Autodesk Inventor part; units mm, degrees
ref_plane "YZ Plane" through (0, 0, 0) normal (1, 0, 0) x (0, 1, 0)
ref_plane "XZ Plane" through (0, 0, 0) normal (0, 1, 0) x (-1, 0, 0)
ref_plane "XY Plane" through (0, 0, 0) normal (0, 0, 1) x (1, 0, 0)
sketch "Sketch1" plane through (0, 0, 0) normal (0, 1, 0) x (-1, 0, 0)
  line L0 (-0.0949, -0.0791) -> (-0.0949, -8.0791)
  circle A0 centre (-0.0949, -8.0791) radius 3
  line L1 (-0.0949, -0.0791) -> (-0.0949, 7.9209)
  circle A1 centre (-0.0949, 7.9209) radius 2.5
  circle A2 centre (-0.0949, 7.9209) radius 3.75
  circle A3 centre (-0.0949, -8.0791) radius 3.75
  line L2 (3.6551, 7.9209) -> (3.6551, -8.0791)
  line L3 (-3.8449, 7.9209) -> (-3.8449, -8.0791)
  line L4 (3.6551, 4.1709) -> (-3.8449, 4.1709)
  line L5 (3.6551, -4.3291) -> (-3.8449, -4.3291)
  point P0 (0, 0)
  dimension "d0" = 8
  dimension "d1" = 6
  dimension "d2" = 8
  dimension "d3" = 5
  dimension "d4" = 7.5
  dimension "d5" = 7.5
extrude "Extrusion1" add sketch "Sketch1" along normal blind 5 contours L1 L4 L2 L5 L0 | L0 L5 L3 L4 L1 | L5 L2 A3 | A3 | A3 L3 L5
sketch "Sketch2" plane through (-3.6551, 0, 4.1709) normal (0, 0, 1) x (1, 0, 0)
  line L0 (0, 5) -> (7.5, 5)
  line L1 (0, 0) -> (7.5, 0)
  line L2 (7.5, 0) -> (7.5, 5)
  line L3 (7.5, 5) -> (0, 5)
  line L4 (0, 5) -> (0, 0)
  line L5 (7.5, 5) -> (0, 5)
  line L6 (0, 5) -> (0, 0)
  line L7 (0, 0) -> (7.5, 0)
  line L8 (7.5, 0) -> (7.5, 5)
  line L9 (7.5, 5) -> (0, 0) construction
  line L10 (0, 5) -> (7.5, 0) construction
  circle A0 centre (3.75, 2.5) radius 1.5
  line L11 (6.25, 3.5) -> (1.25, 3.5)
  line L12 (1.25, 3.5) -> (1.25, 1.5)
  line L13 (1.25, 1.5) -> (6.25, 1.5)
  line L14 (6.25, 1.5) -> (6.25, 3.5)
  line L15 (6.25, 3.5) -> (1.25, 1.5) construction
  line L16 (1.25, 3.5) -> (6.25, 1.5) construction
  point P0 (3.6551, 0)
  point P1 (4.868, 1.5)
  point P2 (4.868, 3.5)
  point P3 (2.632, 3.5)
  point P4 (2.632, 1.5)
  dimension "d8" = 3
  dimension "d9" = 5
  dimension "d10" = 2
extrude "Extrusion2" cut sketch "Sketch2" against normal blind 8.5 contours A0 L13 L11 | A0 L11 L14 L13 | L11 A0 | A0 L13 | A0 L13 L12 L11
sketch "Sketch3" plane through (0, 5, 0) normal (0, 1, 0) x (1, 0, 0)
  line L0 (1.213, 4.3291) -> (2.5949, 4.3291)
  line L1 (-3.6551, -4.1709) -> (3.8449, -4.1709)
  point P0 (0, 0)
  dimension "d13" = 8.5
sketch "Sketch4" plane through (3.8449, 0, 4.1709) normal (1, 0, 0) x (0, 0, -1)
  line L0 (12.25, 0) -> (12.25, 5)
  circle A0 centre (12.25, 2.5) radius 1.5
  point P0 (4.1709, 0)
  dimension "d14" = 3
extrude "Extrusion3" add sketch "Sketch4" along normal mid plane 1.5
sketch "Sketch5" plane through (4.5949, 2.5, -8.0791) normal (1, 0, 0) x (0, 0, -1)
  line L0 (0, -2.5) -> (0, 2.5)
  circle A0 centre (0, 0) radius 1
  point P0 (-8.0791, -2.5)
  dimension "d17" = 2
extrude "Extrusion4" cut sketch "Sketch5" against normal blind 3.0875
properties part number "Link_OutsideV3"
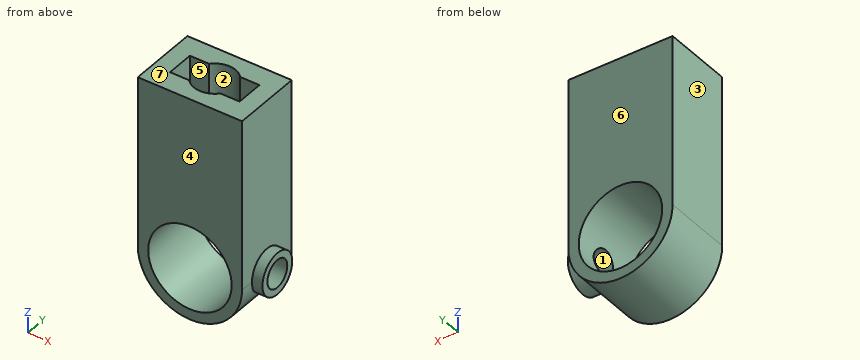
CAD build for the part. Positions are in the model's coordinates, mm. Face numbers are marked on the shaded views. A direction names the side the tool comes from. Coordinates: 2 decimals unless noted, no trailing zeros. Order: outer loops, then holes, each group sorted by start corner. A loop starts at its lowest first (then second) coordinate and runs counter-clockwise, first axis right, second up.
Item 1: Pin check, flat tips, straight feed: pin 1 Ø1.5 at (x, y) = (0.5, 2) entering from +Z; pin 2 Ø1.6 at (y, z) = (3, -1) entering from +X; pin 3 Ø1.5 at (x, z) = (-1.5, -8) entering from +Y. Stop position of each tip, or through.
Check sheet entries:
pin 1: stops at z = -4.33
pin 2: stops at x = 3.84
pin 3: passes through
Item 2: 3-axis set-ups, long thin cutter, end or side, ignore diameter. For the marked faces 1, 2 and 3: which of +Z, -Z, +X, -X, +Y, -Y reach the whole face in a straight line?
Check sheet entries:
face 1: +X
face 2: +Z
face 3: +Z, -Z, -X, +Y, -Y
Item 3: Band-saw the part on B-B on y = 4.35. List the corners of the cut face in (x, z), plus the area to 3 significant figures.
Check sheet entries:
outline: (-3.66, -8.08) arc R3.75 ccw to (3.84, -8.08) - (3.84, 4.17) - (-3.66, 4.17) - close; hole circle Ø6 at (0.09, -8.08)
area: 85.7 mm2
Item 4: Band-saw the part on C-C on x = 0. List the corners of the cut face in (y, z), plus the area to 3 significant figures.
Check sheet entries:
outline: (0, -11.83) - (5, -11.83) - (5, -11.08) - (0, -11.08) - close; (0, -5.08) - (5, -5.08) - (5, 4.17) - (4, 4.17) - (4, -4.33) - (1, -4.33) - (1, 4.17) - (0, 4.17) - close
area: 24.6 mm2
Item 5: Drill centre lines: L1, parallel to X at y = 2.6, z = -2; L2, parallel to Y at x = 2.5, z = -2.5; L3, parallel to Y at x = 0, z = 2. Where is each one in solid material? Low to high.
Check sheet entries:
L1: x = -3.66 to -2.41, 2.59 to 3.84
L2: y = 0 to 1.5, 3.5 to 5
L3: y = 0 to 1, 4 to 5
Item 6: Two-plate mould, pull along Y, no slides. Class the marked faces 4, 5, 6 and 7: +Y half, -Y half, draft (parallel to the pull), parting line (faces both ways), or undercut.
Check sheet entries:
face 4: -Y half
face 5: undercut
face 6: +Y half
face 7: draft
Item 7: Band-saw the part on D-D on y = 2.5. List the corners of the cut face in (x, z).
Check sheet entries:
outline: (-3.66, -8.08) arc R3.75 ccw to (3.53, -9.58) - (4.59, -9.58) - (4.59, -9.08) - (2.92, -9.08) arc R3 cw (long way) to (2.92, -7.08) - (4.59, -7.08) - (4.59, -6.58) - (3.84, -6.58) - (3.84, 4.17) - (2.59, 4.17) - (2.59, -4.33) - (-2.41, -4.33) - (-2.41, 4.17) - (-3.66, 4.17) - close
Item 8: Band-saw the part on A-A on z = -2.5. List the corners of the cut face in (x, y), plus the area to 3 significant figures.
Check sheet entries:
outline: (-3.66, 0) - (3.84, 0) - (3.84, 5) - (-3.66, 5) - close; hole (-2.41, 1.5) - (-1.02, 1.5) arc R1.5 ccw to (1.21, 1.5) - (2.59, 1.5) - (2.59, 3.5) - (1.21, 3.5) arc R1.5 ccw to (-1.02, 3.5) - (-2.41, 3.5) - close
area: 26.0 mm2
